Job drawing, mm, ordinate dimensions from the low corner. One solid piece. A direction names the side the tool comes from. Round coordinates to 2 decimals unless told otherwise and drop trailing zeros. Order: outer loops, then holes, each group sorted by start corner. A loop starts at its lowest first (then second) coordinate and runs counter-clockwise, first axis right, second up. Notation, with made-up numbers: M -21.5,79 L -0.5,79 A4 cw -0.5,85 Z; hole C 89,16.25 d9. An arc over 180 degrees is marked long. Answer as a JSON object with one key per item and string values. Group by question number.
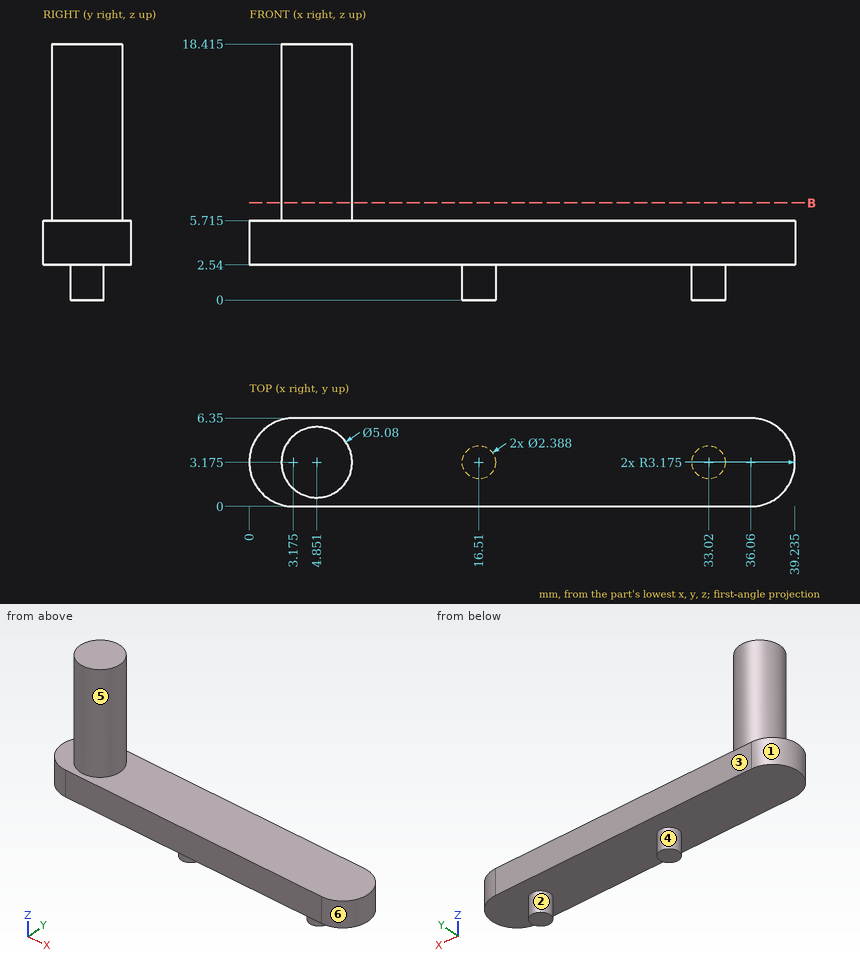
Item 1: Cut at B-B, the plane z = 7. Give the cut face in (x, y) (1 decimal), and give its area (3 significant figures).
Item 2: Drill centre lines: line 1 (Z direction, x = 27, y = 5.5) (1 decimal); line 2 (X direction, y = 3, z = 14.25) (1 decimal); line 3 (X direction, y = 2, z = 13.5). Where is each one in solid material? Low to high. Write a range as [from, to].
Item 3: Flat gauge pin, fed straight in: pin 1 Ø3 at (x, y) = (14, 3.5) entering from +Z (3 decimals). Where does the tip first touch, or does it go through?
Item 4: 3-axis set-ups, long thin cutter, end or side, ignore diameter. For the marked faces 4, 5 and 6: which of +Z, -Z, +X, -X, +Y, -Y reach the whole face in a straight line?
Item 5: Two-plate mould, pull along X, no slides. Class the marked faces 1, 2 and 3: +X half, -X half, draft (parallel to the pull), parting line (faces both ways), or undercut.
Response values:
{
 "1": {"outline": "C 4.9,3.2 d5.1", "area": "20.3 mm^2"},
 "2": {"line 1": "[2.5, 5.7]", "line 2": "[2.3, 7.4]", "line 3": "[2.6, 7.1]"},
 "3": {"pin 1": "z = 5.715"},
 "4": {"face 4": "-Z", "face 5": "+Z", "face 6": "+Z, -Z, +X"},
 "5": {"face 1": "-X half", "face 2": "undercut", "face 3": "draft"}
}
